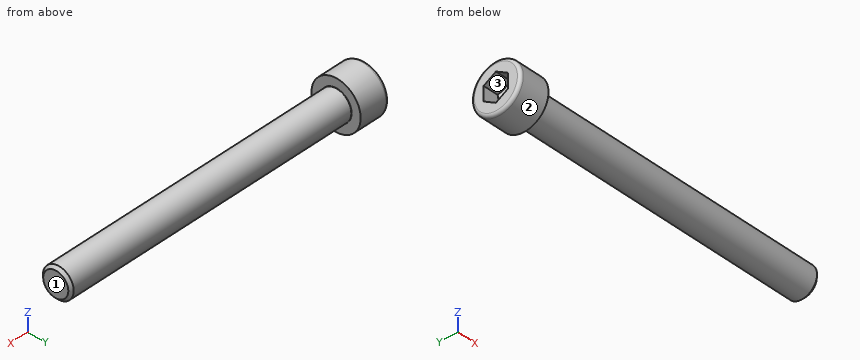
Autodesk Inventor part; units mm, degrees
ref_plane "Work Plane1" through (29, 0, 0) normal (0, -1, 0) x (1, 0, 0)
ref_plane "YZ Plane" through (0, 0, 0) normal (1, 0, 0) x (0, 1, 0)
ref_plane "XZ Plane" through (0, 0, 0) normal (0, 1, 0) x (-1, 0, 0)
sketch "Эскиз1" plane through (0, 0, 0) normal (0, 0, 1) x (1, 0, 0)
  line L0 (-2.3333, 0) -> (100, 0)
  line L1 (100, 0) -> (100, 5)
  line L2 (100, 5) -> (74, 5)
  line L3 (74, 5) -> (73.0797, 5)
  line L4 (73.0797, 5) -> (0, 5)
  line L5 (0, 5) -> (0, 8)
  line L6 (0, 8) -> (-10, 8)
  line L7 (-10, 8) -> (-10, 4.6188)
  line L8 (-10, 4.6188) -> (-5, 4.6188)
  line L9 (-5, 4.6188) -> (-2.3333, 0)
  line L10 (-33, 0) -> (128, 0)
  line L11 (0, -1.6) -> (0, 9.6)
  line L12 (74, 5) -> (0, 5) construction
  dimension "d1" = 26
  dimension "d2" = 0.9203
  dimension "d3" = 10
  dimension "d4" = 5
  dimension "d5" = 60
  dimension "d6" = 10
  dimension "d7" = 10
  dimension "d8" = 9.2376
  dimension "d9" = 16
  dimension "d26" = 100
revolve "Базовый элемент" add sketch "Эскиз1" angle 360 about axis through (-2.3333, 0, 0) along (1, 0, 0)
sketch "Эскиз2" plane through (-10, 0, 0) normal (-1, 0, 0) x (0, 0, 1)
  circle A0 centre (0, 0) radius 4.6188
  line L0 (0, -11.2) -> (0, 11.2)
  line L1 (-11.2, 0) -> (11.2, 0)
  line L2 (4.6188, 0) -> (2.3094, -4)
  line L3 (2.3094, -4) -> (-2.3094, -4)
  line L4 (-2.3094, -4) -> (-4.6188, 0)
  line L5 (-4.6188, 0) -> (-2.3094, 4)
  line L6 (-2.3094, 4) -> (2.3094, 4)
  line L7 (2.3094, 4) -> (4.6188, 0)
extrude "Паз" add sketch "Эскиз2" against normal up to next contours L7 A0 | A0 L2 | L6 L0 A0 | A0 L0 L3 | L0 L6 A0 | A0 L3 L0 | L4 A0 | A0 L5
fillet "Сопряжение1" radius 1 1 edges at (-10, -8, 0)
thread "Резьба"
chamfer "Фаска1" distance 0.9202 distance2 0.9202 1 edges at (100, -5, 0) measured on face at (100, -0.4485, 2.7318)
ref_plane "Work Plane1" through (29, 0, 0) normal (0, -1, 0) x (1, 0, 0)
fillet "Fillet2" radius 0.1 1 edges at (0, -5, 0)
equation "\"d1\" = GEL"
equation "\"d3\" = KOH"
equation "\"d4\" = INTI"
equation "\"d6\" = GD"
equation "\"d7\" = BDM"
equation "\"d8\" = 1.1547 * SW"
equation "\"d9\" = KOD"
equation "\"d26\" = NLG"
equation "\"d30\" = R"
equation "\"d17\" = RR"
equation "\"d13\" = GEL"
equation "\"d15\" = -0.5 * SPD + 0.5 * GD"
equation "\"d16\" = GUL"
equation "\"GD\" = NND"
equation "\"NLG\" = 100"
equation "\"GEL\" = 26"
equation "\"KOD\" = 16"
equation "\"KOH\" = NND"
equation "\"INTI\" = 5"
equation "\"GAL\" = 0.61345 * PTC"
equation "\"GUL\" = 0.61345 * PTC"
equation "\"BDM\" = NND"
equation "\"SW\" = 8"
equation "\"RR\" = 0.1 * NND"
equation "\"SPD\" = NND - 1.2269 * PTC"
equation "\"R\" = 0.1"
equation "\"PHH\" = 0.2"
equation "\"GD1\" = THREADDIA - 1.2269 * PTC"
equation "\"FAWI\" = 45deg"
equation "\"PTC\" = 1.5"
equation "\"KOH1\" = 9"
equation "\"TOA\" = 30deg"
equation "\"E0\" = 1.155 * SW"
properties part number "AS 1420 - 1973 - M10 x 80" material "Сталь, мягкая"
Here's how the part is built. I have some questions about the finished solid (model axes, mm). Face numbers are marked on the shaded views. Give positions to 0.01 mm unless a question says otherwise; leave off trailing zeros. Order: outer loops, then holes, each group sorted by start corner. A loop starts at its lowest first (then second) coordinate and runs counter-clockwise, first axis right, second up. Notation, with made-up numbers: (20, 78) -> (75, 78) arc R15 ccw to (75, 99) -> close; hole circle Ø6 at (82.25, -27.5). An arc over 180 degrees is marked (long way). One line per item, written item: value. Start each with the question number.
1. Imagine slicing it at A-A, the plane x = 26. List the corners of the cut face in (y, z) for me, plus the area to 3 significant figures.
2. I need wall thicknesses on probe 1 along Z at (x, y) = (16, 0.25); probe 2 along X at (y, z) = (5.5, -1.5); probe 3 along Y at (x, z) = (88.5, 3). Which ranges of each line are inside material? Lowest first, please. Write a range as from..to.
3. We'd pull the mould along Z, two halves only. Please class the marked faces 1, 2 and 3: released by +Z, released by -Z, zero draft, split by the parting line, or undercut.
4. Will these pins go through, and if not, where does the flat tip stop? pin 1 Ø1 at (x, y) = (5, -5) entering from +Z; pin 2 Ø6 at (x, z) = (56.5, -5.5) entering from -Y; pin 3 Ø1 at (x, z) = (41.5, -2.5) entering from -Y.
Values follow:
1. outline: circle Ø10 at (0, 0)
1. area: 78.5 mm2
2. probe 1: z = -4.99..4.99
2. probe 2: x = -10..0
2. probe 3: y = -4..4
3. face 1: zero draft
3. face 2: split by the parting line
3. face 3: undercut
4. pin 1: stops at z = 2.18
4. pin 2: stops at y = -4.33
4. pin 3: stops at y = -4.58
